Design review of the part built by this model. Coordinates are the model's own, in mm. A direction names the side the tool comes from. Round coordinates to 2 decimals unless told otherwise and drop trailing zeros. Order: outer loops, then holes, each group sorted by start corner. A loop starts at its lowest first (then second) coordinate and runs counter-clockwise, first axis right, second up. Notation, with made-up numbers: (34, 21.25) - (48, 21.25) arc R19 ccw to (48, 58.25) - close; hole circle Ø9 at (25.25, 53). An arc over 180 degrees is marked (long way). Write item = value, one per line.
from build123d import *

# Parameters (mm, degrees)
SKETCH1_R             = 60
BOSS_EXTRUDE1_DEPTH   = 18
SKETCH2_R             = 12.5
CUT_EXTRUDE1_DEPTH    = 87.740993769
SKETCH3_R             = 6.654092803
CUT_EXTRUDE2_DEPTH    = 12.480181
CIRPATTERN1_START     = 5.519819249
CIRPATTERN1_OUTLINE_R = 6.654092803
CIRPATTERN1_DEPTH     = 12.480180751


# Read off the part's stored shape, not the designer's step: CirPattern1
with BuildPart() as part:
    # Sketch1 → Boss-Extrude1 (new body)
    with BuildSketch(Plane(origin=(0, 0, 0), x_dir=(1, 0, 0), z_dir=(0, 1, 0))):
        with Locations(Location((0, 0, 0), (0, 0, 270))):
            Circle(SKETCH1_R)
    extrude(amount=BOSS_EXTRUDE1_DEPTH)

    # Sketch2 → Cut-Extrude1 (cut, through all)
    with BuildSketch(Plane(origin=(0, 0, 0), x_dir=(1, 0, 0), z_dir=(0, 1, 0))):
        with Locations(Location((0, 0, 0), (0, 0, 270))):
            Circle(SKETCH2_R)
    extrude(amount=CUT_EXTRUDE1_DEPTH, mode=Mode.SUBTRACT)

    # Sketch3 → Cut-Extrude2 (cut)
    with BuildSketch(Plane(origin=(0, 18, 0), x_dir=(1, 0, 0), z_dir=(0, 1, 0))):
        with Locations(Location((-25.242105276, 0, 0), (0, 0, 270))):
            Circle(SKETCH3_R)
    extrude(amount=-CUT_EXTRUDE2_DEPTH, mode=Mode.SUBTRACT)

    # CirPattern1 outline → CirPattern1 (cut)
    with BuildSketch(Plane(origin=(0, 0, 0), x_dir=(1, 0, 0), z_dir=(0, 1, 0)).offset(CIRPATTERN1_START)):
        with Locations((-17.848863812, -17.848863812)):
            Circle(CIRPATTERN1_OUTLINE_R)
        with Locations((-17.848863812, 17.848863812)):
            Circle(CIRPATTERN1_OUTLINE_R)
        with Locations((0, 25.242105276)):
            Circle(CIRPATTERN1_OUTLINE_R)
        with Locations((17.848863812, 17.848863812)):
            Circle(CIRPATTERN1_OUTLINE_R)
        with Locations((25.242105276, 0)):
            Circle(CIRPATTERN1_OUTLINE_R)
        with Locations((17.848863812, -17.848863812)):
            Circle(CIRPATTERN1_OUTLINE_R)
        with Locations((0, -25.242105276)):
            Circle(CIRPATTERN1_OUTLINE_R)
    extrude(amount=CIRPATTERN1_DEPTH, mode=Mode.SUBTRACT)


solid = part.part
1) For faces 5 (the cylindrical face through (3.755, 8.874, 11.923)), 6 (the cylindrical face through (-23.13, 11.67, -13.8)), list the 3-axis set-ups (+Z, -Z, +X, -X, +Y, -Y) from which the entire face can be reached by the end or side of a thin tool; tool diameter is ignored.
Findings:
face_5 = +Y, -Y
face_6 = +Y
2) Clearance check with flat-ended pins moving along their axes: pin 1 Ø10 at (y, z) = (10.5, 33.5) entering from +X; pin 2 Ø15.5 at (x, z) = (0, -25.24) entering from -Y; pin 3 Ø6.5 at (x, z) = (1, -22.5) entering from +Y; pin 4 Ø3 at (y, z) = (4.5, -11) entering from +X. State where each tip first meets the part, or that it passes through.
Findings:
pin_1 = 52.8
pin_2 = 0
pin_3 = 5.52
pin_4 = 59.24
3) The part is to be moulded in two halves that separate along X. For faces 1 (the cylindrical face through (2.64, 8.87, -59.94)), 2 (the flat face through (14, 18, -1)), 3 (the cylindrical face through (-31.145, 11.847, 3.07)), 4 (the cylindrical face through (-1.44, 11.67, 31.74)), say which applies: released by +X, released by -X, zero draft, split by the parting line, or undercut.
Findings:
face_1 = split by the parting line
face_2 = zero draft
face_3 = undercut
face_4 = undercut
4) We need section B-B on x = 0. Write out the cut boundary in (y, z), and give its area (3 significant figures).
Findings:
outline = (0, -60) - (18, -60) - (18, -31.9) - (5.52, -31.9) - (5.52, -18.59) - (18, -18.59) - (18, -12.5) - (0, -12.5) - close; (0, 12.5) - (18, 12.5) - (18, 18.59) - (5.52, 18.59) - (5.52, 31.9) - (18, 31.9) - (18, 60) - (0, 60) - close
area = 1,380 mm^2
5) To check wall thickness, follow L1, parallel to X at y = 6, z = 0; L2, parallel to Z at x = 15, y = 13; L3, parallel to X at y = 10.75, z = -22. State the ranges of each line that lie inside material, in increasing order. Write a range as from..to.
Findings:
L1 = -60..-31.9, -18.59..-12.5, 12.5..18.59, 31.9..60
L2 = -58.09..-23.86, -11.84..11.84, 23.86..58.09
L3 = -55.82..-23.05, -12.65..-5.81, 5.81..12.65, 23.05..55.82
6) We need section D-D on z = 44.5. Write out the cut boundary in (x, y).
Findings:
outline = (-40.25, 0) - (40.25, 0) - (40.25, 18) - (-40.25, 18) - close
7) We need section A-A on z = 0. Write out the cut boundary in (x, y).
Findings:
outline = (-60, 0) - (-12.5, 0) - (-12.5, 18) - (-18.59, 18) - (-18.59, 5.52) - (-31.9, 5.52) - (-31.9, 18) - (-60, 18) - close; (12.5, 0) - (60, 0) - (60, 18) - (31.9, 18) - (31.9, 5.52) - (18.59, 5.52) - (18.59, 18) - (12.5, 18) - close
8) We need section C-C on y = 9.75. Give the number of separate pieces and of enclosed holes in the cut face, and give its area (3 significant figures).
Findings:
separate_pieces = 1
enclosed_holes = 9
area = 9,710 mm^2
